Build history of the part. All positions in model axes, mm. A direction names the side the tool comes from. Round coordinates to 2 decimals unless told otherwise and drop trailing zeros. Write each loop counter-clockwise with the first axis right and the second up, starting at its lowest first coordinate (ties: lowest second). Pieces come first, ordered by that corner, then holes. Notation, with made-up numbers: (32.5, 28) -> (46.5, 28) arc R17 cw to (46.5, 38) -> close; hole circle Ø1 at (-19, 67). An arc over 180 degrees is marked (long way). Answer in a Markdown table with one row per item. Add a question column.
from build123d import *

# Parameters (mm, degrees)
CROQUIS1_R              = 100
SALIENTE_EXTRUIR1_DEPTH = 104
CROQUIS3_R              = 20
CROQUIS2_R              = 100
CROQUIS4_R              = 20
SALIENTE_EXTRUIR2_DEPTH = 65
CROQUIS5_R              = 32.5
SALIENTE_EXTRUIR3_DEPTH = 40
CROQUIS6_R              = 27.5
CORTAR_EXTRUIR1_DEPTH   = 334.803834764
CROQUIS7_R              = 17.5
CORTAR_EXTRUIR2_DEPTH   = 24


with BuildPart() as part:
    # Croquis1 → Saliente-Extruir1 (new body)
    with BuildSketch(Plane(origin=(0, 0, 0), x_dir=(1, 0, 0), z_dir=(0, 1, 0))):
        with Locations(Location((0, 0, 0), (0, 0, 270))):
            Circle(CROQUIS1_R)
    extrude(amount=-SALIENTE_EXTRUIR1_DEPTH)

    # Croquis3 → Recubrir1 section 0
    with BuildSketch(Plane(origin=(0, -230, 0), x_dir=(1, 0, 0), z_dir=(0, 1, 0))):
        Circle(CROQUIS3_R)
    # Croquis2 → Recubrir1 section 1
    with BuildSketch(Plane.XZ.offset(104)):
        Circle(CROQUIS2_R)
    loft()

    # Croquis4 → Saliente-Extruir2 (add)
    with BuildSketch(Plane.XZ.offset(230)):
        with Locations(Location((0, 0, 0), (0, 0, 270))):
            Circle(CROQUIS4_R)
    extrude(amount=SALIENTE_EXTRUIR2_DEPTH)

    # Croquis5 → Saliente-Extruir3 (add)
    with BuildSketch(Plane(origin=(0, 0, -20), x_dir=(-1, 0, 0), z_dir=(0, 0, -1))):
        with Locations((0, -262.5)):
            Circle(CROQUIS5_R)
    extrude(amount=-SALIENTE_EXTRUIR3_DEPTH)

    # Croquis6 → Cortar-Extruir1 (cut, through all)
    with BuildSketch(Plane(origin=(0, 0, -20), x_dir=(-1, 0, 0), z_dir=(0, 0, -1))):
        with Locations((0, -262.5)):
            Circle(CROQUIS6_R)
    extrude(amount=-CORTAR_EXTRUIR1_DEPTH, mode=Mode.SUBTRACT)

    # Croquis7 → Cortar-Extruir2 (cut)
    with BuildSketch(Plane.XZ.offset(295)):
        with Locations(Location((0, 0, 0), (0, 0, 270))):
            Circle(CROQUIS7_R)
    extrude(amount=-CORTAR_EXTRUIR2_DEPTH, mode=Mode.SUBTRACT)


solid = part.part
(1) Saw through at A-A (y = -262.5). List the corners of the cut face in (x, z), plus the area to 3 significant figures.
(2) Saw through at C-C (x = 7). Count the separate pieces of the cut face and the enclosed holes in it, plus the area to 3 significant figures.
(3) Mould opens along X. For faces 1 (the face through (-17.084, -290.689, 3.794)), 2 (the face through (-18, -295, 0)), 3 (the face through (-20, -233, 0)) say: pulls with the +X half, pulls with the -X half, needs draft (parallel to the pull), parting line crosses it, or undercut.
(4) Saw through at B-B (y = -100). List the corners of the cut face in (x, z), plus the area to 3 significant figures.
(5) Drop flat-ended pins along their axis: P1, Ø3, axis at x = -69, y = -158.5, coming from the +Z side; P2, Ø6, axis at x = 63, y = -88.5, coming from the +Z side; P3, Ø2, axis at x = 31.5, y = -162, coming from the +Z side; P4, Ø4, axis at x = 49, y = -118, coming from the +Z side. Give the stop position or say it passes through.
(6) Probe line 1 along X through (y, z) = (-262, -11); line 2 along X through (y, z) = (-290.25, 0); line 3 along Y through (x, z) = (-17, -13.5). List the from-to ranges inside material, lowest first.
(7) Which spindle directions (+Z, -Z, +X, -X, +Y, -Y) get a long thin tool onto all of the face, cutting with end or side? Do faces 4 (the face through (-20, -292, 0)), 5 (the face through (20, -233, 0)), 6 (the face through (27, -255, -20)), 7 (the face through (20, -292, 0)). Say none if no direction does.
Answer sheet:
| question | item | result |
|---|---|---|
| 1 | outline | (-32.5, -20) -> (-27.5, -20) -> (-27.5, 20) -> (-32.5, 20) -> close; (27.5, -20) -> (32.5, -20) -> (32.5, 20) -> (27.5, 20) -> close |
| 1 | area | 400 mm² |
| 2 | separate pieces | 3 |
| 2 | enclosed holes | 0 |
| 2 | area | 36,000 mm² |
| 3 | face 1 | undercut |
| 3 | face 2 | needs draft |
| 3 | face 3 | pulls with the -X half |
| 4 | outline | circle Ø200 at (0, 0) |
| 4 | area | 31,400 mm² |
| 5 | P1 | passes through |
| 5 | P2 | stops at z = 80 |
| 5 | P3 | stops at z = 55.68 |
| 5 | P4 | stops at z = 78.76 |
| 6 | line 1 | x = -32.5 to -27.5, 27.5 to 32.5 |
| 6 | line 2 | x = -20 to -17.5, 17.5 to 20 |
| 6 | line 3 | y = -290.2 to -284.12, -240.88 to -234.8, -227.31 to 0 |
| 7 | face 4 | -X, -Y |
| 7 | face 5 | +X |
| 7 | face 6 | -Z, +X, -X, -Y |
| 7 | face 7 | +X, -Y |
